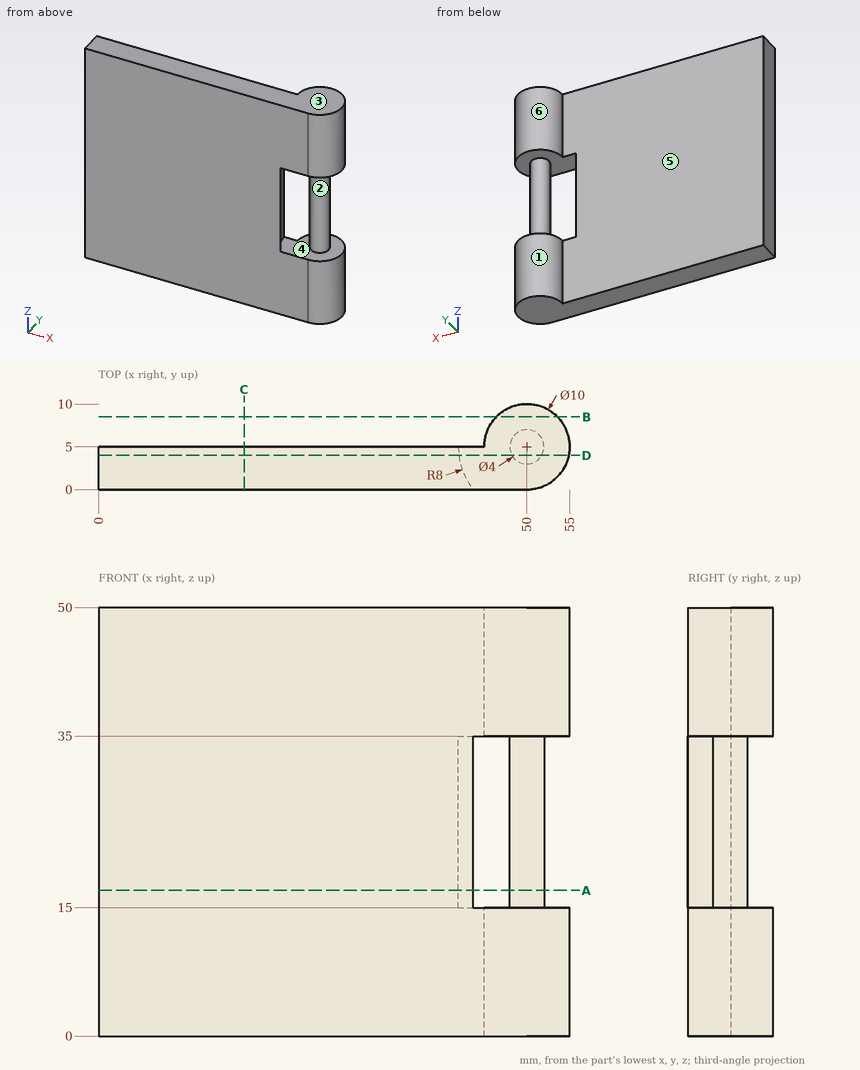
Drawing for the job (mm, zero at the part's lowest x, y, z). A direction names the side the tool comes from. Round coordinates to 2 decimals unless told otherwise and drop trailing zeros. Loops run counter-clockwise (first coordinate to the right, second up) from the corner with the lowest first, then second, coordinate; pieces in that order, holes last. Notation, with made-up numbers: (80, 76) - (128, 76) arc R29 ccw to (128, 106) - close; hole circle Ø2 at (88.5, 59). An arc over 180 degrees is marked (long way). Return JSON: item names as keys, results as strings. Group by question number.
Q1. Band-saw the part on D-D on y = 4. Give the cut face in (x, z).
Q2. Band-saw the part on C-C on x = 17. Give the cut face in (y, z).
Q3. Two-plate mould, pull along Z, no slides. Class the marked faces 1, 2 and 3: +Z half, -Z half, draft (parallel to the pull), parting line (faces both ways), or undercut.
Q4. Band-saw the part on A-A on z = 17. Give the cut face in (x, y) (3 decimals), plus the area to 3 significant figures.
Q5. Tool access for the marked faces 4, 5 and 6: list every direction of +Z, -Z, +X, -X, +Y, -Y with a clear straight run to the whole face (end or side of a thin tool).
Q6. Flat gauge pins, fed straight in: pin 1 Ø13.5 at (x, z) = (32, 27.5) entering from +Y; pin 2 Ø4 at (x, y) = (7.5, 8) entering from +Z. Where does each tip first touch, or does it go through?
Q7. Band-saw the part on B-B on y = 8.5. Give the cut face in (x, z).
Q8. Drill centre lines: line 1 along Z through (x, y) = (47.5, 3.5); line 2 along Y through (x, z) = (41.5, 24.5); line 3 along X through (y, z) = (3.5, 34.5). Where is each one in solid material? Low to high. Write a range as [from, to].
Solutions:
{
 "1": {"outline": "(0, 0) - (54.9, 0) - (54.9, 15) - (51.73, 15) - (51.73, 35) - (54.9, 35) - (54.9, 50) - (0, 50) - close; hole (42.06, 15) - (48.27, 15) - (48.27, 35) - (42.06, 35) - close"},
 "2": {"outline": "(0, 0) - (5, 0) - (5, 50) - (0, 50) - close"},
 "3": {"face 1": "draft", "face 2": "undercut", "face 3": "+Z half"},
 "4": {"outline": "(0, 0) - (43.755, 0) arc R8 cw to (42, 5) - (0, 5) - close; circle Ø4 at (50, 5)", "area": "225 mm^2"},
 "5": {"face 4": "none", "face 5": "+Z, -Z, -X, +Y", "face 6": "+Z, -Z"},
 "6": {"pin 1": "stops at y = 5", "pin 2": "passes through"},
 "7": {"outline": "(46.43, 0) - (53.57, 0) - (53.57, 15) - (46.43, 15) - close; (46.43, 35) - (53.57, 35) - (53.57, 50) - (46.43, 50) - close"},
 "8": {"line 1": "z = [0, 15], [35, 50]", "line 2": "y = [0, 5]", "line 3": "x = [0, 42.14], [48.68, 51.32]"}
}
